from build123d import *

# Parameters (mm, degrees)
SKETCH1_W                    = 191.7
SKETCH1_H                    = 99.64
BASE_FLANGE4_DEPTH           = 2
EDGE_FLANGE2_STRIP_W         = 11.175
EDGE_FLANGE2_STRIP_H         = 2
EDGE_FLANGE2_STRIP_CUT_DEPTH = 191.7
EDGE_FLANGE2_DEPTH           = 191.7
EDGE_FLANGE1_START           = -49.82
EDGE_FLANGE1_DEPTH           = 99.64
EDGE_FLANGE1_START_2         = 46.2325
EDGE_FLANGE1_2_DEPTH         = 3.5875
EDGE_FLANGE1_3_DEPTH         = 96.0525
EDGE_FLANGE3_START           = -97.85
EDGE_FLANGE3_DEPTH           = 195.7
EDGE_FLANGE3_2_DEPTH         = 3.5875
EDGE_FLANGE3_START_2         = 94.2625
EDGE_FLANGE3_3_DEPTH         = 3.5875
EDGE_FLANGE3_START_3         = -94.2625
EDGE_FLANGE3_4_DEPTH         = 188.525
CUT_EXTRUDE1_DEPTH           = 204.46180182
CUT_EXTRUDE2_DEPTH           = 3.175


# Read off the part's stored shape, not the designer's step: Edge-Flange1, Edge-Flange3
# Sheet-metal steps are written as plain solids
with BuildPart() as part:
    # Sketch1 → Base-Flange4 (new body)
    with BuildSketch(Plane.XY):
        Rectangle(SKETCH1_W, SKETCH1_H)
    extrude(amount=-BASE_FLANGE4_DEPTH)

    # Edge-Flange2 strip (across the edge) → Edge-Flange2 strip cut (cut)
    with BuildSketch(Plane(origin=(95.85, 49.82, 0), x_dir=(0, -1, 0), z_dir=(-1, 0, 0))):
        with Locations((-2, -1)):
            Rectangle(EDGE_FLANGE2_STRIP_W, EDGE_FLANGE2_STRIP_H)
    extrude(amount=EDGE_FLANGE2_STRIP_CUT_DEPTH, mode=Mode.SUBTRACT)

    # Edge-Flange2 section (across the edge) → Edge-Flange2 (add)
    with BuildSketch(Plane(origin=(95.85, 49.82, 0), x_dir=(0, -1, 0), z_dir=(-1, 0, 0))):
        with BuildLine():
            Line((0, 1.5875), (0, 10.7))
            Line((0, 10.7), (2, 10.7))
            Line((2, 10.7), (2, 1.5875))
            ThreePointArc((2, 1.5875), (2.464967985, 0.464967985), (3.5875, 0))
            Line((3.5875, 0), (3.5875, -2))
            ThreePointArc((3.5875, -2), (1.050754422, -0.949245578), (0, 1.5875))
        make_face()
    extrude(amount=EDGE_FLANGE2_DEPTH)

    # Edge-Flange1 outline → Edge-Flange1 (cut)
    with BuildSketch(Plane(origin=(0, 0, 0), x_dir=(1, 0, 0), z_dir=(0, 1, 0)).offset(EDGE_FLANGE1_START)):
        with BuildLine():
            Line((94.2625, -1.5875), (95.85, -1.5875))
            Line((95.85, -1.5875), (95.85, 0.370358411))
            ThreePointArc((95.85, 0.370358411), (95.07756466, 0.093816292), (94.2625, 0))
            Line((94.2625, 0), (94.2625, -1.5875))
        make_face()
        with BuildLine():
            Line((-95.85, 0.370358411), (-95.85, -1.5875))
            Line((-95.85, -1.5875), (-94.2625, -1.5875))
            Line((-94.2625, -1.5875), (-94.2625, 0))
            ThreePointArc((-94.2625, 0), (-95.07756466, 0.093816292), (-95.85, 0.370358411))
        make_face()
    extrude(amount=EDGE_FLANGE1_DEPTH, mode=Mode.SUBTRACT)

    # Edge-Flange1 2 outline → Edge-Flange1 2 (cut)
    with BuildSketch(Plane(origin=(0, 0, 0), x_dir=(1, 0, 0), z_dir=(0, 1, 0)).offset(EDGE_FLANGE1_START_2)):
        with BuildLine():
            Line((94.2625, 2), (94.2625, 0))
            ThreePointArc((94.2625, 0), (95.07756466, 0.093816292), (95.85, 0.370358411))
            ThreePointArc((95.85, 0.370358411), (97.30924519, 1.693430307), (97.85, 3.5875))
            Line((97.85, 3.5875), (97.85, 20.32))
            Line((97.85, 20.32), (95.85, 20.32))
            Line((95.85, 20.32), (95.85, 3.5875))
            ThreePointArc((95.85, 3.5875), (95.385032015, 2.464967985), (94.2625, 2))
        make_face()
        with BuildLine():
            ThreePointArc((-95.85, 0.370358411), (-95.07756466, 0.093816292), (-94.2625, 0))
            Line((-94.2625, 0), (-94.2625, 2))
            ThreePointArc((-94.2625, 2), (-95.385032015, 2.464967985), (-95.85, 3.5875))
            Line((-95.85, 3.5875), (-95.85, 20.32))
            Line((-95.85, 20.32), (-97.85, 20.32))
            Line((-97.85, 20.32), (-97.85, 3.5875))
            ThreePointArc((-97.85, 3.5875), (-97.30924519, 1.693430307), (-95.85, 0.370358411))
        make_face()
    extrude(amount=EDGE_FLANGE1_2_DEPTH, mode=Mode.SUBTRACT)

    # Edge-Flange1 3 outline → Edge-Flange1 3 (add)
    with BuildSketch(Plane(origin=(0, 0, 0), x_dir=(1, 0, 0), z_dir=(0, 1, 0)).offset(EDGE_FLANGE1_START)):
        with BuildLine():
            Line((94.2625, 2), (94.2625, 0))
            ThreePointArc((94.2625, 0), (95.07756466, 0.093816292), (95.85, 0.370358411))
            ThreePointArc((95.85, 0.370358411), (97.30924519, 1.693430307), (97.85, 3.5875))
            Line((97.85, 3.5875), (97.85, 20.32))
            Line((97.85, 20.32), (95.85, 20.32))
            Line((95.85, 20.32), (95.85, 3.5875))
            ThreePointArc((95.85, 3.5875), (95.385032015, 2.464967985), (94.2625, 2))
        make_face()
        with BuildLine():
            ThreePointArc((-95.85, 0.370358411), (-95.07756466, 0.093816292), (-94.2625, 0))
            Line((-94.2625, 0), (-94.2625, 2))
            ThreePointArc((-94.2625, 2), (-95.385032015, 2.464967985), (-95.85, 3.5875))
            Line((-95.85, 3.5875), (-95.85, 20.32))
            Line((-95.85, 20.32), (-97.85, 20.32))
            Line((-97.85, 20.32), (-97.85, 3.5875))
            ThreePointArc((-97.85, 3.5875), (-97.30924519, 1.693430307), (-95.85, 0.370358411))
        make_face()
    extrude(amount=EDGE_FLANGE1_3_DEPTH)

    # Edge-Flange3 outline → Edge-Flange3 (cut)
    with BuildSketch(Plane.YZ.offset(EDGE_FLANGE3_START)):
        with BuildLine():
            ThreePointArc((-48.2325, -2), (-49.355032015, -2.464967985), (-49.82, -3.5875))
            Line((-49.82, -3.5875), (-48.2325, -3.5875))
            Line((-48.2325, -3.5875), (-48.2325, -2))
        make_face()
        with BuildLine():
            ThreePointArc((-49.82, -0.370358411), (-49.04756466, -0.093816292), (-48.2325, 0))
            Line((-48.2325, 0), (-49.82, 0))
            Line((-49.82, 0), (-49.82, -0.370358411))
        make_face()
    extrude(amount=EDGE_FLANGE3_DEPTH, mode=Mode.SUBTRACT)

    # Edge-Flange3 2 outline → Edge-Flange3 2 (cut)
    with BuildSketch(Plane.YZ.offset(EDGE_FLANGE3_START)):
        with BuildLine():
            ThreePointArc((-49.82, -3.5875), (-49.355032015, -2.464967985), (-48.2325, -2))
            Line((-48.2325, -2), (-48.2325, 0))
            ThreePointArc((-48.2325, 0), (-49.04756466, -0.093816292), (-49.82, -0.370358411))
            Line((-49.82, -0.370358411), (-49.82, -3.5875))
        make_face()
    extrude(amount=EDGE_FLANGE3_2_DEPTH, mode=Mode.SUBTRACT)

    # Edge-Flange3 3 outline → Edge-Flange3 3 (cut)
    with BuildSketch(Plane.YZ.offset(EDGE_FLANGE3_START_2)):
        with BuildLine():
            ThreePointArc((-49.82, -3.5875), (-49.355032015, -2.464967985), (-48.2325, -2))
            Line((-48.2325, -2), (-48.2325, 0))
            ThreePointArc((-48.2325, 0), (-49.04756466, -0.093816292), (-49.82, -0.370358411))
            Line((-49.82, -0.370358411), (-49.82, -3.5875))
        make_face()
    extrude(amount=EDGE_FLANGE3_3_DEPTH, mode=Mode.SUBTRACT)

    # Edge-Flange3 4 outline → Edge-Flange3 4 (add)
    with BuildSketch(Plane.YZ.offset(EDGE_FLANGE3_START_3)):
        with BuildLine():
            Line((-48.2325, -2), (-49.82, -2))
            Line((-49.82, -2), (-49.82, -0.370358411))
            ThreePointArc((-49.82, -0.370358411), (-51.27924519, -1.693430307), (-51.82, -3.5875))
            Line((-51.82, -3.5875), (-51.82, -20.32))
            Line((-51.82, -20.32), (-49.82, -20.32))
            Line((-49.82, -20.32), (-49.82, -3.5875))
            ThreePointArc((-49.82, -3.5875), (-49.355032015, -2.464967985), (-48.2325, -2))
        make_face()
    extrude(amount=EDGE_FLANGE3_4_DEPTH)

    # Sketch42 → Cut-Extrude1 (cut, through all)
    with BuildSketch(Plane.ZY.offset(97.85)):
        with BuildLine():
            ThreePointArc((-9.566529979, 34.815400328), (-12.586590694, 37.822400713), (-15.593591079, 34.802339997))
            Line((-15.593591079, 34.802339997), (-15.61375, 33.5325))
            Line((-15.61375, 33.5325), (-15.61375, 32.2625))
            ThreePointArc((-15.61375, 32.2625), (-12.58875, 29.2375), (-9.56375, 32.2625))
            Line((-9.56375, 32.2625), (-9.56375, 33.5325))
            Line((-9.56375, 33.5325), (-9.566529979, 34.815400328))
        make_face()
        with BuildLine():
            Line((-15.61375, -35.85), (-15.61375, -38.39))
            ThreePointArc((-15.61375, -38.39), (-12.58875, -41.415), (-9.56375, -38.39))
            Line((-9.56375, -38.39), (-9.56375, -35.85))
            ThreePointArc((-9.56375, -35.85), (-12.58875, -32.825), (-15.61375, -35.85))
        make_face()
        with BuildLine():
            Line((-9.56375, -3.2975), (-9.56375, -2.0275))
            Line((-9.56375, -2.0275), (-9.566529979, -0.744599672))
            ThreePointArc((-9.566529979, -0.744599672), (-12.586590694, 2.262400713), (-15.593591079, -0.757660003))
            Line((-15.593591079, -0.757660003), (-15.61375, -2.0275))
            Line((-15.61375, -2.0275), (-15.61375, -3.2975))
            ThreePointArc((-15.61375, -3.2975), (-12.58875, -6.3225), (-9.56375, -3.2975))
        make_face()
    extrude(amount=-CUT_EXTRUDE1_DEPTH, mode=Mode.SUBTRACT)

    # Sketch43 → Cut-Extrude2 (cut)
    with BuildSketch(Plane.XZ.offset(51.82)):
        with BuildLine():
            Line((-23.1425, -8.92875), (-25.6825, -8.92875))
            ThreePointArc((-25.6825, -8.92875), (-28.448425456, -12.005254825), (-25.572047177, -14.97875))
            Line((-25.572047177, -14.97875), (-23.1425, -14.97875))
            ThreePointArc((-23.1425, -14.97875), (-20.1175, -11.95375), (-23.1425, -8.92875))
        make_face()
        with BuildLine():
            Line((34.0075, -8.92875), (31.4675, -8.92875))
            ThreePointArc((31.4675, -8.92875), (28.701574544, -12.005254825), (31.577952823, -14.97875))
            Line((31.577952823, -14.97875), (34.0075, -14.97875))
            ThreePointArc((34.0075, -14.97875), (37.0325, -11.95375), (34.0075, -8.92875))
        make_face()
        with BuildLine():
            ThreePointArc((-80.2925, -14.97875), (-77.2675, -11.95375), (-80.2925, -8.92875))
            Line((-80.2925, -8.92875), (-82.8325, -8.92875))
            ThreePointArc((-82.8325, -8.92875), (-85.598425456, -12.005254825), (-82.722047177, -14.97875))
            Line((-82.722047177, -14.97875), (-80.2925, -14.97875))
        make_face()
        with BuildLine():
            Line((82.2675, -8.92875), (79.7275, -8.92875))
            ThreePointArc((79.7275, -8.92875), (76.961574544, -12.005254825), (79.837952823, -14.97875))
            Line((79.837952823, -14.97875), (82.2675, -14.97875))
            ThreePointArc((82.2675, -14.97875), (85.2925, -11.95375), (82.2675, -8.92875))
        make_face()
    extrude(amount=-CUT_EXTRUDE2_DEPTH, mode=Mode.SUBTRACT)


solid = part.part
Source: CAD feature listing. Evaluate the final solid. Frame: model axes, mm. A direction names the side the tool comes from. Give positions to 0.01 mm unless a question says otherwise; leave off trailing zeros. Order: outer loops, then holes, each group sorted by start corner. A loop starts at its lowest first (then second) coordinate and runs counter-clockwise, first axis right, second up. Notation, with made-up numbers: (80.25, 30) -> (111.25, 30) arc R18 cw to (111.25, 59) -> close; hole circle Ø9 at (-20.75, 21.25). An arc over 180 degrees is marked (long way). Write item = value, one per line.
Q1. Pull-direction query (X, two-part tool) for faces 6 (the face through (-97, 46.232, -10)), 7 (the face through (-1, -49.82, -12)), 8 (the face through (94.262, 48, 0)); classes: released by +X, released by -X, zero draft, split by the parting line, or undercut.
Data:
face_6 = zero draft
face_7 = undercut
face_8 = released by +X
Q2. Set-up query: faces 1 (the face through (96, -48.232, -2)), 2 (the face through (-94.262, -51, -10)), 3 (the face through (1, 47.82, 6)), 4 (the face through (97, 46.232, -10)), 5 (the face through (-95.85, -2, -8)). Return all of +Z, -Z, +X, -X, +Y, -Y with unobstructed straight access to the full face (end or side cutting, diameter ignored); none if empty.
Data:
face_1 = +Z, +X, -Y
face_2 = +Z, -Z, -X, -Y
face_3 = +Z, +X, -X, -Y
face_4 = +Z, -Z, +X, +Y
face_5 = -Z, +Y, -Y
Q3. Material intervals for line 1 (X direction, y = -9, z = -9); line 2 (Y direction, x = 59, z = -9.5); line 3 (Y direction, x = 14.5, z = 3.5), sorted ascending. Write a range as from..to.
Data:
line_1 = -97.85..-95.85, 95.85..97.85
line_2 = -51.82..-49.82
line_3 = 47.82..49.82
Q4. Pin query (flat end, axial travel): pin 1 (4 mm diameter, centred on y = -0.5, z = -1, fed in from +X); pin 2 (0.6 mm diameter, centred on y = 49.5, z = 5.5, fed in from +X); pin 3 (8 mm diameter, centred on x = -32, y = 23, fed in from +Z). Return the tip coordinate at first contact, or that it passes through.
Data:
pin_1 = 97.8
pin_2 = 95.85
pin_3 = 0
Q5. Cut plane A-A, the plane x = 44. Output: boundary loops of the cut face in (y, z) (1 decimal), and give its area (3 significant figures).
Data:
outline = (-51.8, -20.3) -> (-49.8, -20.3) -> (-49.8, -3.6) arc R1.6 cw to (-48.2, -2) -> (46.2, -2) arc R3.6 ccw to (49.8, 1.6) -> (49.8, 10.7) -> (47.8, 10.7) -> (47.8, 1.6) arc R1.6 cw to (46.2, 0) -> (-48.2, 0) arc R3.6 ccw to (-51.8, -3.6) -> close
area = 257 mm^2
Q6. Cut plane C-C, the plane z = 5. Output: boundary loops of the cut face in (x, y), and give its area (3 significant figures).
Data:
outline = (-95.85, 47.82) -> (95.85, 47.82) -> (95.85, 49.82) -> (-95.85, 49.82) -> close
area = 383 mm^2
